Could you check a few things on this model? Use its own coordinates, in mm. A direction names the side the tool comes from. Round coordinates to 2 decimals unless told otherwise and drop trailing zeros. Write each loop counter-clockwise with the first axis right and the second up, starting at its lowest first coordinate (ties: lowest second). Pieces come first, ordered by that corner, then holes. Notation, with made-up numbers: (18, 73) - (24, 73) arc R28 ccw to (24, 111) - close; hole circle Ø10 at (22, 33.5). An arc over 180 degrees is marked (long way). Write each question's results on one line, items separated by ' | '. Start each with the question number.
(1) On a 3-axis mill with a long thin cutter (end or side, diameter ignored), from which of +Z, -Z, +X, -X, +Y, -Y can I reach the whole of each face in a straight line? I mean faces 1 (the conical face through (0.591, 0.844, -1.623)), 2 (the cylindrical face through (5, 0, -1)). Say none if no direction works.
(2) For P1, Ø0.5, axis at x = 0.5, z = -1, coming from the +Y side; P2, Ø2, axis at x = 3.5, y = 0, coming from the +Z side; P3, Ø0.7, axis at x = 0.5, z = -1, coming from the -Y side, each with a flat end and sliding along its axis, tell me the tip position at first contact or that it passes through.
(3) Please list where these lines run through material, in increasing order: line 1 (Z direction, x = 2, y = -0.05); line 2 (Y direction, x = 0.5, z = -1.3); line 3 (X direction, y = 0.05, z = 0.15). Write a range as [from, to].
(4) Imagine slicing it at B-B on z = 0. Write out the boundary of the cut face in (x, y).
(5) Imagine slicing it at A-A on y = 0. Write out the boundary of the cut face in (x, z), then the cut area to 3 significant figures.
(6) Imagine slicing it at C-C on x = 4.75. Write out the boundary of the cut face in (y, z), then the cut area to 3 significant figures.
(7) Imagine slicing it at D-D on x = 1.25. Write out the boundary of the cut face in (y, z).
```python
from build123d import *

# Parameters (mm, degrees)
FILLET2_R  = 0.1
SKETCH2_W  = 3.8
SKETCH2_H  = 0.5
SLOT_DEPTH = 0.6


with BuildPart() as part:
    # BodySke → Base-Revolve (revolve)
    with BuildSketch(Plane.XY):
        Polygon((1.4, 1), (1.4, 1.9), (0, 1.777515871), (0, 0), (9.4, 0), (9.4, 1), align=None)
    revolve(axis=Axis((-25.4, 0, 0), (1, 0, 0)))

    # Fillet2
    fillet2_edges = [part.edges().sort_by_distance(p)[0] for p in [
        (0, -1.777515871, 0),
    ]]
    fillet(fillet2_edges, radius=FILLET2_R)

    # Sketch2 → Slot (cut)
    with BuildSketch(Plane(origin=(0, 0, 0), x_dir=(0, 0, -1), z_dir=(1, 0, 0))):
        Rectangle(SKETCH2_W, SKETCH2_H)
    extrude(amount=SLOT_DEPTH, mode=Mode.SUBTRACT)


solid = part.part
```
Response:
1) face 1: -X | face 2: +X
2) P1: y = 1.66 | P2: z = 1 | P3: y = -1.71
3) line 1: [-1, 1] | line 2: [-1.28, -0.25], [0.25, 1.28] | line 3: [0.6, 9.4]
4) outline: (0, -1.69) arc R0.1 ccw to (0.09, -1.79) - (1.4, -1.9) - (1.4, -1) - (9.4, -1) - (9.4, 1) - (1.4, 1) - (1.4, 1.9) - (0.09, 1.79) arc R0.1 ccw to (0, 1.69) - (0, 0.25) - (0.6, 0.25) - (0.6, -0.25) - (0, -0.25) - close
5) outline: (0.6, -1.83) - (1.4, -1.9) - (1.4, -1) - (9.4, -1) - (9.4, 1) - (1.4, 1) - (1.4, 1.9) - (0.6, 1.83) - close | area: 19.0 mm²
6) outline: circle Ø2 at (0, 0) | area: 3.14 mm²
7) outline: circle Ø3.77 at (0, 0)
